Read the model definition and answer for the solid it produces. Units are mm, in the model's axes. Give positions to 0.01 mm unless a question says otherwise; leave off trailing zeros. Loops run counter-clockwise (first coordinate to the right, second up) from the corner with the lowest first, then second, coordinate; pieces in that order, holes last. Notation, with made-up numbers: (34, 43.5) -> (73, 43.5) arc R27 ccw to (73, 68.5) -> close; hole circle Ø10 at (26.5, 16). An arc over 180 degrees is marked (long way). Return JSON: item names as keys, results as strings. Group by question number.
from build123d import *

# Parameters (mm, degrees)
CROQUIS1_R              = 4
SALIENTE_EXTRUIR1_DEPTH = 1.5
CROQUIS3_R              = 2.5
CROQUIS3_W              = 20
CROQUIS3_H              = 2.8
CROQUIS3_W_2            = 25
CORTAR_EXTRUIR2_DEPTH   = 3


with BuildPart() as part:
    # Croquis1 → Saliente-Extruir1 (new, symmetric)
    with BuildSketch(Plane(origin=(0, 0, 0), x_dir=(1, 0, 0), z_dir=(0, 1, 0))):
        Polygon((-77, -42), (-77, -54), (77, -54), (77, -42), (74, -42), (74, -28), (77, -28), (77, -20), (74, -20), (74, -12), (77, -12), (77, -4), (74, -4), (74, -1.5), (74, 1.5), (74, 4), (77, 4), (77, 12), (74, 12), (74, 14.497912952), (70.25, 14.497912952), (70.25, 12), (67.25, 12), (67.25, 14.497912952), (66.27, 14.497912952), (66.27, 17.992083938), (67.25, 17.992083938), (67.25, 20), (70.25, 20), (70.25, 17.992083938), (74, 17.992083938), (74, 20), (77, 20), (77, 28), (74, 28), (74, 42), (77, 42), (77, 54), (65, 54), (65, 51), (55, 51), (55, 54), (45, 54), (45, 51), (31.5, 51), (31.5, 47.25), (34, 47.25), (34, 44.25), (31.5, 44.25), (31.5, 43.27), (28.5, 43.27), (28.5, 44.25), (26, 44.25), (26, 47.25), (28.5, 47.25), (28.5, 51), (15, 51), (15, 54), (5, 54), (5, 51), (-5, 51), (-5, 54), (-15, 54), (-15, 51), (-28.5, 51), (-28.5, 47.25), (-26, 47.25), (-26, 44.25), (-28.5, 44.25), (-28.5, 43.27), (-31.5, 43.27), (-31.5, 44.25), (-34, 44.25), (-34, 47.25), (-31.5, 47.25), (-31.5, 51), (-45, 51), (-45, 54), (-55, 54), (-55, 51), (-65, 51), (-65, 54), (-77, 54), (-77, 42), (-74, 42), (-74, 28), (-77, 28), (-77, 20), (-74, 20), (-74, 17.992083938), (-70.25, 17.992083938), (-70.25, 20), (-67.25, 20), (-67.25, 17.992083938), (-66.27, 17.992083938), (-66.27, 14.497912952), (-67.25, 14.497912952), (-67.25, 12), (-70.25, 12), (-70.25, 14.497912952), (-74, 14.497912952), (-74, 12), (-77, 12), (-77, 4), (-74, 4), (-74, 1.5), (-74, -1.5), (-74, -4), (-77, -4), (-77, -12), (-74, -12), (-74, -20), (-77, -20), (-77, -28), (-74, -28), (-74, -42), align=None)
        with Locations(Location((-65, -48, 0), (0, 0, 270))):
            Circle(CROQUIS1_R, mode=Mode.SUBTRACT)
        with BuildLine():
            Line((55, -49.6), (53, -49.6))
            ThreePointArc((53, -49.6), (52.646446609, -49.453553391), (52.5, -49.1))
            Line((52.5, -49.1), (52.5, -46.4))
            Line((52.5, -46.4), (55.5, -46.4))
            Line((55.5, -46.4), (55.5, -49.1))
            ThreePointArc((55.5, -49.1), (55.353553391, -49.453553391), (55, -49.6))
        make_face(mode=Mode.SUBTRACT)
    extrude(amount=SALIENTE_EXTRUIR1_DEPTH, both=True)

    # Croquis3 → Cortar-Extruir2 (cut)
    with BuildSketch(Plane(origin=(0, 1.5, 0), x_dir=(1, 0, 0), z_dir=(0, 1, 0))):
        with Locations(Location((-19.5, 33.79, 0), (0, 0, 270))):
            Circle(CROQUIS3_R)
        with Locations(Location((19.5, 33.79, 0), (0, 0, 270))):
            Circle(CROQUIS3_R)
        with Locations((0, 12.9)):
            Rectangle(CROQUIS3_W, CROQUIS3_H)
        with Locations((0, -12.9)):
            Rectangle(CROQUIS3_W, CROQUIS3_H)
        with Locations((0, -23.4)):
            Rectangle(CROQUIS3_W_2, CROQUIS3_H)
    extrude(amount=-CORTAR_EXTRUIR2_DEPTH, mode=Mode.SUBTRACT)


solid = part.part
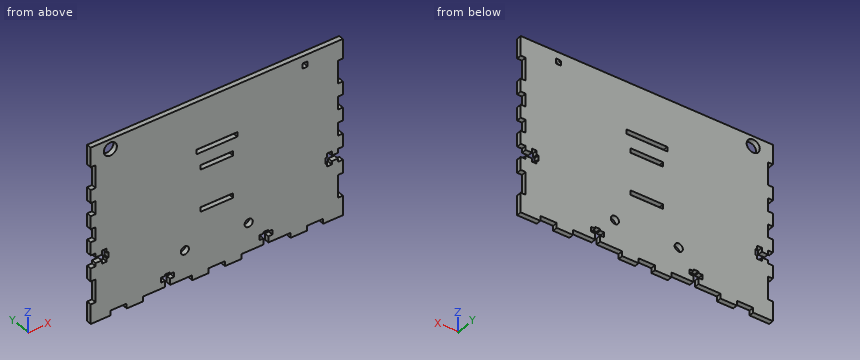
1. Section C-C on x = -19.5 is taken. Determine the outline of the cut face in (y, z).
2. Flat-ended cylindrical pins translate along their axes: pin 1 Ø1.4 at (y, z) = (0, -13) entering from -X; pin 2 Ø0.9 at (y, z) = (-0.5, -17) entering from -X. Find the tip coordinate at first contact, or state that the pin passes through.
3. Section B-B on z = -33.79 is taken. Determine the outline of the cut face in (x, y).
4. Section D-D on y = -0.95 is taken. State how many separate pieces and enclosed holes the cut face has, then the cut area to 3 significant figures.
5. Section A-A on x = 0.5 is taken. Determine the outline of the cut face in (y, z).
6. Straight lines are drawn through the part: line 1 (X direction, y = 0, z = -33.79); line 2 (Z direction, x = -9, y = 1.2); line 3 (X direction, y = -0.35, z = 48). For each, find the intervals that lie inside material, in ascending order. Write a range as from..to.
Completed:
{
 "1": {"outline": "(-1.5, -51) -> (1.5, -51) -> (1.5, -36.29) -> (-1.5, -36.29) -> close; (-1.5, -31.29) -> (1.5, -31.29) -> (1.5, 54) -> (-1.5, 54) -> close"},
 "2": {"pin 1": "stops at x = -74", "pin 2": "stops at x = -66.27"},
 "3": {"outline": "(-74, -1.5) -> (-22, -1.5) -> (-22, 1.5) -> (-74, 1.5) -> close; (-17, -1.5) -> (17, -1.5) -> (17, 1.5) -> (-17, 1.5) -> close; (22, -1.5) -> (74, -1.5) -> (74, 1.5) -> (22, 1.5) -> close"},
 "4": {"separate pieces": "1", "enclosed holes": "7", "area": "15,600 mm²"},
 "5": {"outline": "(-1.5, -51) -> (1.5, -51) -> (1.5, -14.3) -> (-1.5, -14.3) -> close; (-1.5, -11.5) -> (1.5, -11.5) -> (1.5, 11.5) -> (-1.5, 11.5) -> close; (-1.5, 14.3) -> (1.5, 14.3) -> (1.5, 22) -> (-1.5, 22) -> close; (-1.5, 24.8) -> (1.5, 24.8) -> (1.5, 54) -> (-1.5, 54) -> close"},
 "6": {"line 1": "x = -74..-22, -17..17, 22..74", "line 2": "z = -54..-14.3, -11.5..11.5, 14.3..22, 24.8..54", "line 3": "x = -77..-69, -61..52.5, 55.5..77"}
}
